Input: part model. Units: mm. Frame: model coordinates. A direction names the side the tool comes from. Give positions to 0.01 mm unless a question says otherwise; leave off trailing zeros. Loops run counter-clockwise (first coordinate to the right, second up) from the corner with the lowest first, then second, coordinate; pieces in that order, holes last. Notation, with made-up numbers: (80, -32) -> (92, -32) arc R24 ccw to (92, -21) -> close; hole circle Ø11 at (-18, 89.5). An arc over 180 degrees is marked (long way). One line per question, with ' | ' between items.
from build123d import *
from build123d.topology import SkipClean

# Parameters (mm, degrees)
SKETCH1_W           = 280
SKETCH1_H           = 280
SKETCH1_R           = 16
BOSS_EXTRUDE1_DEPTH = 1.5
SKETCH2_R           = 7.5
SKETCH2_W           = 4
SKETCH2_H           = 73.713198053
SKETCH2_W_2         = 58
SKETCH2_H_2         = 4
SKETCH2_H_3         = 64
SKETCH2_W_3         = 32
SKETCH2_H_4         = 34
BOSS_EXTRUDE2_DEPTH = 7


with BuildPart() as part:
    # Sketch1 → Boss-Extrude1 (new, symmetric)
    with BuildSketch(Plane(origin=(0, 0, 0), x_dir=(1, 0, 0), z_dir=(0, 1, 0))):
        Rectangle(SKETCH1_W, SKETCH1_H)
        with Locations(Location((-96, 103, 0), (0, 0, 270))):
            Circle(SKETCH1_R, mode=Mode.SUBTRACT)
    extrude(amount=BOSS_EXTRUDE1_DEPTH, both=True)

    # Sketch2 → Boss-Extrude2 (add)
    with SkipClean():  # the faces are left unmerged after this step: merging them gives an invalid solid
        with BuildSketch(Plane(origin=(0, 1.5, 0), x_dir=(1, 0, 0), z_dir=(0, 1, 0))):
            with Locations(Location((-54.759044634, 52.982810669, 0), (0, 0, 270))):
                Circle(SKETCH2_R)
            with Locations(Location((-89.473504534, 19.023832923, 0), (0, 0, 270))):
                Circle(SKETCH2_R)
            with Locations(Location((-83.738928303, -33.690548853, 0), (0, 0, 270))):
                Circle(SKETCH2_R)
            with Locations(Location((-109.516269096, -61.269929812, 0), (0, 0, 270))):
                Circle(SKETCH2_R)
            with Locations(Location((-80.69273369, -98.230062392, 0), (0, 0, 270))):
                Circle(SKETCH2_R)
            with Locations(Location((37.587423323, -55.831973409, 0), (0, 0, 270))):
                Circle(SKETCH2_R)
            with Locations(Location((105.9104653, -70.333190482, 0), (0, 0, 270))):
                Circle(SKETCH2_R)
            with Locations(Location((11.819316554, -7.352500668, 0), (0, 0, 270))):
                Circle(SKETCH2_R)
            with Locations(Location((-9.755931913, 39.066973306, 0), (0, 0, 270))):
                Circle(SKETCH2_R)
            with Locations(Location((29.170109307, 94.80128466, 0), (0, 0, 270))):
                Circle(SKETCH2_R)
            with Locations(Location((82.624857116, 73.284632448, 0), (0, 0, 270))):
                Circle(SKETCH2_R)
            with Locations(Location((37.587423323, 33.266850719, 0), (0, 0, 270))):
                Circle(SKETCH2_R)
            with Locations(Location((106.252694304, 33.287862382, 0), (0, 0, 270))):
                Circle(SKETCH2_R)
            with Locations((-49, 103.143400974)):
                Rectangle(SKETCH2_W, SKETCH2_H)
            with BuildLine():
                Line((-94, 140), (-98, 140))
                Line((-98, 140), (-98, 118.874507866))
                ThreePointArc((-98, 118.874507866), (-96, 119), (-94, 118.874507866))
                Line((-94, 118.874507866), (-94, 140))
            make_face()
            with BuildLine():
                Line((-140, 38.624379655), (-98, 38.624379655))
                Line((-98, 38.624379655), (-98, 87.125492134))
                ThreePointArc((-98, 87.125492134), (-96, 87), (-94, 87.125492134))
                Line((-94, 87.125492134), (-94, 38.624379655))
                Line((-94, 38.624379655), (-82, 38.624379655))
                Line((-82, 38.624379655), (-82, 34.624379655))
                Line((-82, 34.624379655), (-140, 34.624379655))
                Line((-140, 34.624379655), (-140, 38.624379655))
            make_face()
            Polygon((-140, -100.418377476), (-96.668523278, -100.418377476), (-96.668523278, -88.738640334), (-92.668523278, -88.738640334), (-92.668523278, -140), (-96.668523278, -140), (-96.668523278, -104.418377476), (-140, -104.418377476), align=None)
            with Locations((-111, 1.423286191)):
                Rectangle(SKETCH2_W_2, SKETCH2_H_2)
            Polygon((-47.345115434, -140), (-47.345115434, -90.364557891), (-71.881878867, -90.364557891), (-71.881878867, -86.364557891), (-47.345115434, -86.364557891), (-47.345115434, -63.088559208), (-43.345115434, -63.088559208), (-43.345115434, -100.418377476), (48.027751829, -100.418377476), (48.027751829, -64.371939455), (52.027751829, -64.371939455), (52.027751829, -100.418377476), (69.827851451, -100.418377476), (69.827851451, -104.418377476), (-43.345115434, -104.418377476), (-43.345115434, -140), align=None)
            Polygon((140, 7.737266613), (81.293142587, 7.737266613), (81.293142587, -29.543544834), (112.431248518, -29.543544834), (112.431248518, -59.777272974), (108.431248518, -59.777272974), (108.431248518, -33.543544834), (77.293142587, -33.543544834), (77.293142587, -7.47679166), (52.027751829, -7.47679166), (52.027751829, -3.47679166), (77.293142587, -3.47679166), (77.293142587, 11.737266613), (140, 11.737266613), align=None)
            with Locations((93.622601552, -108)):
                Rectangle(SKETCH2_W, SKETCH2_H_3)
            Polygon((-99.510735812, -32.111868954), (-95.510735812, -32.111868954), (-95.510735812, -68.594238703), (-99.510735812, -68.594238703), (-99.510735812, -49.675826938), (-114.127069846, -49.675826938), (-114.127069846, -45.675826938), (-99.510735812, -45.675826938), align=None)
            with Locations((124, 46.843999527)):
                Rectangle(SKETCH2_W_3, SKETCH2_H_2)
            Polygon((-73.435195895, -53.042459291), (-69.435195895, -53.042459291), (-69.435195895, -27.528186601), (-11.837088751, -27.528186601), (-11.837088751, -76.919702569), (-7.837088751, -76.919702569), (-7.837088751, -23.528186601), (-53.440050937, -23.528186601), (-53.440050937, 4.043094912), (-36.882667743, 4.043094912), (-36.882667743, 8.043094912), (-53.440050937, 8.043094912), (-53.440050937, 38.63118777), (-57.440050937, 38.63118777), (-57.440050937, -23.528186601), (-73.435195895, -23.528186601), align=None)
            Polygon((114.833141636, 94.80128466), (114.833141636, 90.80128466), (94.203549623, 90.80128466), (94.203549623, 79.625492134), (90.203549623, 79.625492134), (90.203549623, 94.80128466), align=None)
            with Locations((1.57904958, 15.009472223)):
                Rectangle(SKETCH2_W, SKETCH2_H_4)
            Polygon((68.742119222, 71), (68.742119222, 59.19860167), (47.447056499, 59.19860167), (47.447056499, 42.554658178), (51.447056499, 42.554658178), (51.447056499, 55.19860167), (72.742119222, 55.19860167), (72.742119222, 71), align=None)
            Polygon((21.727135977, -46.6315684), (25.727135977, -46.6315684), (25.727135977, -38.844500644), (41.459511743, -38.844500644), (41.459511743, -34.844500644), (25.727135977, -34.844500644), (25.727135977, 66.420221849), (-20.87255933, 66.420221849), (-20.87255933, 116.344219933), (-24.87255933, 116.344219933), (-24.87255933, 34.358038326), (-20.87255933, 34.358038326), (-20.87255933, 62.420221849), (21.727135977, 62.420221849), align=None)
            Polygon((140, 116.845058218), (44.841725693, 116.845058218), (44.841725693, 87.65657302), (40.841725693, 87.65657302), (40.841725693, 105.182034885), (9.848778982, 105.182034885), (9.848778982, 140), (13.848778982, 140), (13.848778982, 109.182034885), (40.841725693, 109.182034885), (40.841725693, 120.845058218), (140, 120.845058218), align=None)
        extrude(amount=BOSS_EXTRUDE2_DEPTH)


solid = part.part
1. Reachability of faces 1 (the flat face through (91.623, 5, 108)), 2 (the flat face through (13.849, 5, -125)), 3 (the flat face through (105, 5, -90.801)), 4 (the flat face through (-11.837, 5, 52)), 5 (the flat face through (-65, 5, 23.528)) from +Z, -Z, +X, -X, +Y, -Y: full face, straight path, thin tool, end or side. Return the list, or none.
Determined:
face 1: +Z, +Y | face 2: -Z, +Y | face 3: +X, +Y | face 4: +Y | face 5: -X, +Y
2. Section query A-A (x = 120.5). Output: boundary loops of the cut face in (y, z).
Determined:
outline: (-1.5, -140) -> (1.5, -140) -> (1.5, -120.85) -> (8.5, -120.85) -> (8.5, -116.85) -> (1.5, -116.85) -> (1.5, -48.84) -> (8.5, -48.84) -> (8.5, -44.84) -> (1.5, -44.84) -> (1.5, -11.74) -> (8.5, -11.74) -> (8.5, -7.74) -> (1.5, -7.74) -> (1.5, 140) -> (-1.5, 140) -> close
3. Section query B-B (y = 4). Count the separate pieces of the cut face and the enclosed holes in it, then the cut area to 3 significant figures.
Determined:
separate pieces: 29 | enclosed holes: 0 | area: 9,180 mm2
4. Ray query, line 1 along X through (y, z) = (7, 112.5); line 2 along Z through (x, y) = (-96, -0.35); line 3 along Z through (x, y) = (-36.5, 5.5). Return the intervals inside material, ascending. Write a range as from..to.
Determined:
line 1: x = -96.67..-92.67, -47.35..-43.35, 91.62..95.62 | line 2: z = -140..-119, -87..140 | line 3: z = 23.53..27.53, 100.42..104.42
5. Pin query (flat end, axial travel): P1, Ø3, axis at x = 24.5, y = 4.5, coming from the +Z side; P2, Ø4.5, axis at y = 5, z = 87.5, coming from the -X side; P3, Ø2, axis at y = 5.5, z = 102.5, coming from the +X side. Return the tip coordinate at first contact, or that it passes through.
Determined:
P1: stops at z = 104.42 | P2: stops at x = -96.67 | P3: stops at x = 95.62
